Autodesk Inventor part; units mm, degrees
ref_plane "YZ Plane" through (0, 0, 0) normal (1, 0, 0) x (0, 1, 0)
ref_plane "XZ Plane" through (0, 0, 0) normal (0, 1, 0) x (-1, 0, 0)
ref_plane "XY Plane" through (0, 0, 0) normal (0, 0, 1) x (1, 0, 0)
sketch "Эскиз1" plane through (0, 0, 0) normal (0, 1, 0) x (-1, 0, 0)
  line L0 (4.0742, 9.2484) -> (4.0742, 7.7484)
  line L1 (4.0742, 7.7484) -> (3.8742, 7.7484)
  line L2 (3.8742, 7.7484) -> (3.8742, 3.7484)
  line L3 (3.8742, 3.7484) -> (4.0742, 3.7484)
  line L4 (4.0742, 3.7484) -> (4.0742, 2.2484)
  line L5 (4.0742, 2.2484) -> (2.5742, 2.2484)
  line L6 (2.5742, 2.2484) -> (2.5742, 9.2484)
  line L7 (2.5742, 9.2484) -> (4.0742, 9.2484)
  point P0 (0, 0)
  dimension "d0" = 1.5
  dimension "d1" = 0.2
  dimension "d2" = 4
  dimension "d3" = 0.2
  dimension "d4" = 1.5
  dimension "d5" = 1.5
  dimension "d6" = 7
revolve "Вращение1" add sketch "Эскиз1" angle 360 about axis through (-2.5742, 0, 2.2484) along (0, 0, 1)
sketch "Эскиз2" plane through (-2.5742, 0, 9.2484) normal (0, 0, 1) x (1, 0, 0)
  circle A0 centre (0, 0) radius 1.3
  circle A1 centre (0, 0) radius 0.35
  circle A2 centre (-6.8053, 0) radius 0.3139
  point P0 (2.5742, 0)
  dimension "d8" = 0.7
sketch "Эскиз3" plane through (-2.5742, 0, 2.2484) normal (0, 0, -1) x (-1, 0, 0)
  circle A0 centre (0, 0) radius 0.35
  point P0 (-2.5742, 0)
  dimension "d9" = 0.7
sketch3d "3D эскиз1"
  line L0 (-2.5742, 0, 2.2484) -> (-2.5742, 0, 1.7484)
  arc A0 (-2.5742, 0, 1.7484) -> (-2.5742, -2, -0.2516) centre (-2.5742, -2, 1.7484) ccw
  dimension "d10" = 2.5
  dimension "d11" = 2
  dimension "d16" = 2
sweep "Сдвиг2" add profiles "Эскиз3" path "3D эскиз1"
sketch3d "3D эскиз2"
  line L0 (-2.5742, 0, 9.2484) -> (-2.5742, 0, 9.7484)
  arc A0 (-2.5742, 0, 9.7484) -> (-2.5742, -2, 11.7484) centre (-2.5742, -2, 9.7484) ccw
  dimension "d12" = 2.5
  dimension "d13" = 2
  dimension "d19" = 2
sweep "Сдвиг3" add profiles "Эскиз2" path "3D эскиз2" contours A1
equation "\"D22\" = d10 + d6 + d12"
The listing builds one solid part. Answer for the finished solid, in the listing's coordinates (mm). Coordinates: 2 decimals unless noted, no trailing zeros. Write each loop counter-clockwise with the first axis right and the second up, starting at its lowest first coordinate (ties: lowest second). Pieces come first, ordered by that corner, then holes. Notation, with made-up numbers: (-21, 55) - (-3, 55) arc R22 ccw to (-3, 94) - close; hole circle Ø3 at (52.25, 63.5). An arc over 180 degrees is marked (long way). Return JSON: item names as keys, results as strings. Group by question number.
Q1. Flat-ended cylindrical pins translate along their axes: pin 1 Ø1.5 at (x, y) = (-3, 0.5) entering from -Z; pin 2 Ø1 at (x, z) = (-3.5, 2) entering from -Y; pin 3 Ø1.5 at (x, y) = (-2, -0.5) entering from -Z. Find the tip coordinate at first contact, or state that the pin passes through.
Q2. The part is cut by section D-D on z = 8. Write down the section's boundary in (x, y), and give its area (3 significant figures).
Q3. The part is cut by section B-B on z = 5.25. Write down the section's boundary in (x, y).
Q4. The part is cut by section C-C on x = -3.4. Write down the section's boundary in (y, z).
Q5. Find the intervals of material crossed by line 1 along Z through (x, y) = (-3.3, 1.15); line 2 along Y through (x, z) = (-2.55, 5); line 3 along Z through (x, y) = (-2.1, -0.6), in increasing order. Write a range as [from, to].
Q6. The part is cut by section A-A on x = -1.8. Write down the section's boundary in (y, z).
Evaluation:
{
 "1": {"pin 1": "stops at z = 0.29", "pin 2": "stops at y = -1.42", "pin 3": "stops at z = -0.4"},
 "2": {"outline": "circle Ø3 at (-2.57, 0)", "area": "7.07 mm2"},
 "3": {"outline": "circle Ø2.6 at (-2.57, 0)"},
 "4": {"outline": "(-1.25, 2.25) - (1.25, 2.25) - (1.25, 3.75) - (1, 3.75) - (1, 7.75) - (1.25, 7.75) - (1.25, 9.25) - (-1.25, 9.25) - (-1.25, 7.75) - (-1, 7.75) - (-1, 3.75) - (-1.25, 3.75) - close"},
 "5": {"line 1": "z = [2.25, 3.75], [7.75, 9.25]", "line 2": "y = [-1.3, 1.3]", "line 3": "z = [2.25, 9.25]"},
 "6": {"outline": "(-1.28, 2.25) - (1.28, 2.25) - (1.28, 3.75) - (1.04, 3.75) - (1.04, 7.75) - (1.28, 7.75) - (1.28, 9.25) - (-1.28, 9.25) - (-1.28, 7.75) - (-1.04, 7.75) - (-1.04, 3.75) - (-1.28, 3.75) - close"}
}
